Design review of the part shown in the three views and the two pictorial views. Dimensions are in mm from the part's minimum x, y and z. A direction names the side the tool comes from. Give positions to 0.01 mm unless a question says otherwise; leave off trailing zeros. Loops run counter-clockwise (first coordinate to the right, second up) from the corner with the lowest first, then second, coordinate; pieces in that order, holes last.
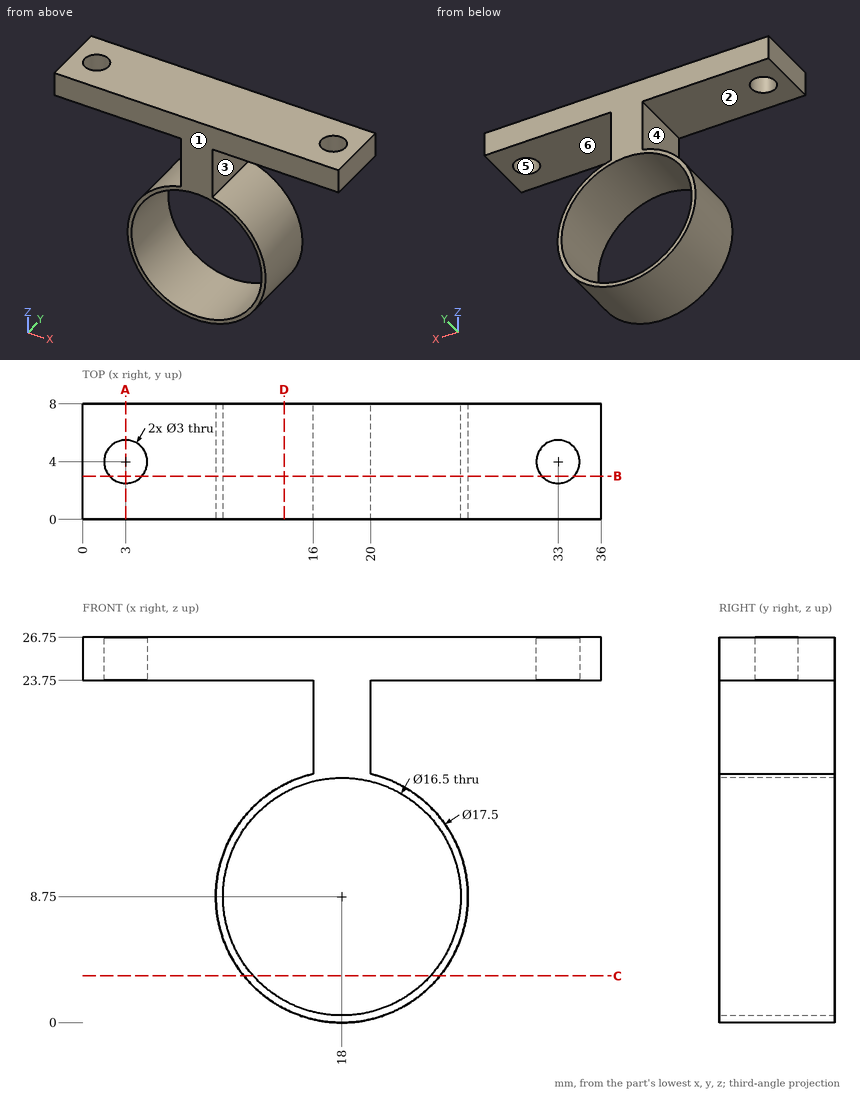
Q1. Take a section at C-C (z = 3.25). Give the boundary of the cut face in (x, y), plus the area to 3 significant figures.
Results:
outline: (11.19, 0) - (11.85, 0) - (11.85, 8) - (11.19, 8) - close; (24.15, 0) - (24.81, 0) - (24.81, 8) - (24.15, 8) - close
area: 10.5 mm2
Q2. Tool access review of the marked faces 1, 2 and 3: name each direction out of +Z, -Z, +X, -X, +Y, -Y from which nothing blocks a thin tool from reaching the whole face with its end or side.
Results:
face 1: +Z, -Z, +X, -X, -Y
face 2: -X, +Y, -Y
face 3: +X, +Y, -Y
Q3. Take a section at B-B (y = 3). Give the boundary of the cut face in (x, z), plus the area to 3 significant figures.
Results:
outline: (0, 23.75) - (1.88, 23.75) - (1.88, 26.75) - (0, 26.75) - close; (4.12, 23.75) - (16, 23.75) - (16, 17.27) arc R8.75 ccw (long way) to (20, 17.27) - (20, 23.75) - (31.88, 23.75) - (31.88, 26.75) - (4.12, 26.75) - close; (34.12, 23.75) - (36, 23.75) - (36, 26.75) - (34.12, 26.75) - close; hole circle Ø16.5 at (18, 8.75)
area: 147 mm2
Q4. Wall thickness on line 1 (Z direction, x = 18, y = 4); line 2 (Z direction, x = 15, y = 6.25); line 3 (Y direction, x = 33, z = 25): over which ranges is each line inside the solid? List them lowest first.
Results:
line 1: z = 0 to 0.5, 17 to 26.75
line 2: z = 0.53 to 1.06, 16.44 to 16.97, 23.75 to 26.75
line 3: y = 0 to 2.5, 5.5 to 8
Q5. Take a section at A-A (x = 3). Give the boundary of the cut face in (y, z), plus the area to 3 significant figures.
Results:
outline: (0, 23.75) - (2.5, 23.75) - (2.5, 26.75) - (0, 26.75) - close; (5.5, 23.75) - (8, 23.75) - (8, 26.75) - (5.5, 26.75) - close
area: 15.0 mm2
Q6. Draft analysis for pull direction X (two halves, no side actions). For the marked faces 4, 5 and 6, state which applies: pulls with the +X half, pulls with the -X half, needs draft (parallel to the pull), parting line crosses it, or undercut.
Results:
face 4: pulls with the -X half
face 5: undercut
face 6: needs draft
Q7. Take a section at D-D (x = 14). Give the boundary of the cut face in (y, z), plus the area to 3 significant figures.
Results:
outline: (0, 0.97) - (8, 0.97) - (8, 1.53) - (0, 1.53) - close; (0, 15.97) - (8, 15.97) - (8, 16.53) - (0, 16.53) - close; (0, 23.75) - (8, 23.75) - (8, 26.75) - (0, 26.75) - close
area: 33.1 mm2
Q8. Insertion check: pin 1 (6 mm diameter, centred on x = 29.5, z = 16, fed in from +Y) (1 decimal); pin 2 (3 mm diameter, centred on y = 5.5, z = 20, fed in from +X); pin 3 (1 mm diameter, centred on y = 5.5, z = 3, fed in from +X); pin 4 (3 mm diameter, centred on y = 3.5, z = 7, fed in from -X). Each pin has a flat end and moves straight along its axis. Give the tip position at first contact, or say it passes through.
Results:
pin 1: passes through
pin 2: stops at x = 20
pin 3: stops at x = 25
pin 4: stops at x = 9.25
